from build123d import *

# Parameters (mm, degrees)
F4_W     = 51.4225922525
F4_H     = 7.856229553
F5_DEPTH = 26


# Not quite as in the source:
# - a feature names something its author has since deleted; it is built from what else it names


with BuildPart() as f1:
    # F0 (on Front) → F1 (revolve)
    with BuildSketch(Plane.XZ):
        with BuildLine():
            Line((22.3186584817, 4.9634656969), (15.2303930372, 1.2544910423))
            Line((15.2303930372, 1.2544910423), (15.488850391, 0.9470738952))
            Line((15.488850391, 0.9470738952), (15.5328564546, 0.894731726))
            Line((15.5328564546, 0.894731726), (15.8405525238, 1.0429841968))
            Line((15.8405525238, 1.0429841968), (22.4313864066, 4.2185444515))
            ThreePointArc((22.4313864066, 4.2185444515), (24.744105662, 3.4097946744), (23.9353558848, 1.097075419))
            Line((23.9353558848, 1.097075419), (16.3696151821, 0.4137007552))
            Line((16.3696151821, 0.4137007552), (15.9677918852, 0.3774061119))
            Line((15.9677918852, 0.3774061119), (16.2850916386, 0))
            Line((16.2850916386, 0), (24.2850916386, 0))
            ThreePointArc((24.2850916386, 0), (25.023915829, 0.2087553322), (25.5442474517, 0.7732860891))
            Line((25.5442474517, 0.7732860891), (25.5442474517, 4.3952541752))
            ThreePointArc((25.5442474517, 4.3952541752), (24.028202675, 5.2285828576), (22.3186584817, 4.9634656969))
        make_face()
        Polygon((15.8405525238, 1.0429841968), (15.5328564546, 0.894731726), (15.9677918852, 0.3774061119), (16.3696151821, 0.4137007552), align=None)
    revolve(axis=Axis((0, 0, 1.8443568842), (0, 0, 1)))

    # F2 (on Front) → F3 (revolve)
    with BuildSketch(Plane.XZ):
        Polygon((-25.3970567137, 3.7070766557), (-28.3970567137, 3.7070766557), (-28.3970567137, 4.2962685693), (-30.5454257131, 3.7070766557), (-30.5454257131, 3.2924627885), (-25.5454257131, 3.2924627885), align=None)
    revolve(axis=Axis((-26.2971473858, 0, 2.2924627885), (-1, 0, 0)))

    # F4 (on Right) → F5 (cut)
    with BuildSketch(Plane.YZ):
        with Locations((-0.0007599592, 2.6581416605)):
            Rectangle(F4_W, F4_H)
    extrude(amount=F5_DEPTH, mode=Mode.SUBTRACT)


solid = f1.part
Check sheet for the modelled part. Datum: model origin and axes. Units: mm. A direction names the side the tool comes from. Give positions to 0.01 mm unless a question says otherwise; leave off trailing zeros. Answer as CSV lines item,"result".
1. Mould release check, pull along X, two halves, no side actions. Record for faces 1 (the face through (-30.545, 1, 3)), 2 (the face through (-28.01, -0.976, 2.076)), 3 (the face through (-28.397, 0, 4)): released by +X, released by -X, zero draft, split by the parting line, or undercut.
Result sheet:
face 1,"released by -X"
face 2,"zero draft"
face 3,"undercut"
2. Tool access check on faces 4 (the face through (-26.97, 0.06, 0.88)), 5 (the face through (-15.571, 0.342, 1.435)). Record the directions out of +Z, -Z, +X, -X, +Y, -Y that give a thin tool (end or side, any length) a straight path to the whole face; none if there is none.
Result sheet:
face 4,"none"
face 5,"+Z, +X"
3. Go/stop test with flat-tipped pins: P1, Ø4, axis at x = -22.5, y = 5, coming from the +Z side; P2, Ø1.2, axis at y = 0.5, z = 2, coming from the +X side; P3, Ø8, axis at x = -6.5, y = -16.5, coming from the +Z side; P4, Ø1.5, axis at x = -27.5, z = 1.5, coming from the -Y side. Record where each tip stops, or that it passes through.
Result sheet:
P1,"z = 5.27"
P2,"x = -15.5"
P3,"z = 4.66"
P4,"y = -1.41"
4. Scan lines: probe 1 along Y at (x, z) = (-8.5, 4.15); probe 2 along Y at (x, z) = (-6, 1.8); probe 3 along X at (y, z) = (2, 4.05). Record each from-to range of solid material in increasing order. Write a range as from..to.
Result sheet:
probe 1,"-24.09..-22.51, -20.6..-18.94, 18.94..20.6, 22.51..24.09"
probe 2,"-24.83..-23.95, -16.35..-15.13, 15.13..16.35, 23.95..24.83"
probe 3,"-25.47..-24.13, -21.99..-20.48"
5. Section check A-A (x = -7). State how many separate pieces and enclosed holes the cut face has, then the cut area to 3 significant figures.
Result sheet:
separate pieces,"2"
enclosed holes,"2"
area,"37.1 mm²"
